Design review of the part built by this model. Coordinates are the model's own, in mm. Coordinates: 2 decimals unless noted, no trailing zeros. Write each loop counter-clockwise with the first axis right and the second up, starting at its lowest first coordinate (ties: lowest second). Pieces come first, ordered by that corner, then holes.
Q1. Take a section at A-A (y = 0). Give the boundary of the cut face in (x, z) (3 decimals), and give its area (3 significant figures).
Q2. For probe 1 along Z at (x, y) = (4.1, 0) (3 decimals); probe 2 along Y at (x, z) = (-1.75, 5.5); probe 3 along Y at (x, z) = (-0.5, 5), list the stretches that pass through material, from the lowest coordinate up.
Q3. Take a section at B-B (z = 9.25). Give the boundary of the cut face in (x, y), and give its area (3 significant figures).
Q4. Insertion check: pin 1 (4 mm diameter, centred on y = 0, z = 6.39, fed in from -X); pin 2 (2 mm diameter, centred on x = -0.5, z = 2.5, fed in from -Y); pin 3 (0.7 mm diameter, centred on x = -0.5, z = 11, fed in from +Y). Each pin has a flat end and moves straight along its axis. Give the tip position at first contact, or say it passes through.
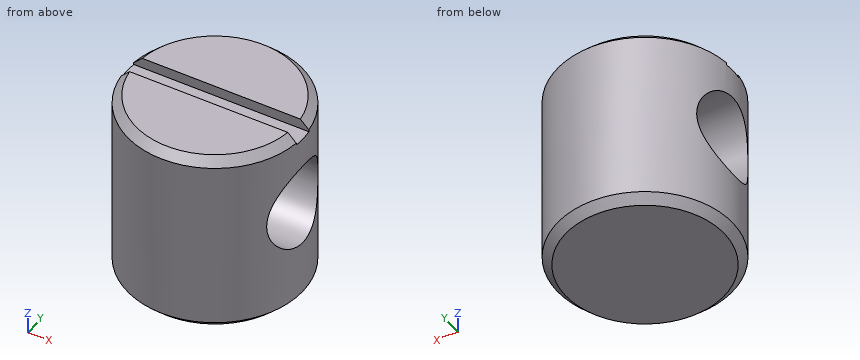
```python
from build123d import *

# Parameters (mm, degrees)
F0_R          = 5.357813
F1_DEPTH      = 11.43
F2_R          = 2.579688
F3_DEPTH      = 25.4
F3_DEPTH_BACK = 25.4
F5_DEPTH      = 0.635
F6_SIZE       = 0.508


with BuildPart() as f1:
    # F0 (on Top) → F1 (new body)
    with BuildSketch(Plane.XY):
        Circle(F0_R)
    extrude(amount=F1_DEPTH)

    # F2 (on Right) → F3 (cut, two sides)
    with BuildSketch(Plane.YZ) as f3_sk:
        with Locations((0, 6.389687)):
            Circle(F2_R)
    extrude(amount=F3_DEPTH, mode=Mode.SUBTRACT)
    extrude(f3_sk.sketch, amount=-F3_DEPTH_BACK, mode=Mode.SUBTRACT)

    # F4 (on face) → F5 (cut)
    with BuildSketch(Plane.XY.offset(11.43)):
        with BuildLine():
            Line((5.32005, 0.635), (-5.32005, 0.635))
            ThreePointArc((-5.32005, 0.635), (-5.379818, 0), (-5.32005, -0.635))
            Line((-5.32005, -0.635), (5.32005, -0.635))
            ThreePointArc((5.32005, -0.635), (5.379818, 0), (5.32005, 0.635))
        make_face()
    extrude(amount=-F5_DEPTH, mode=Mode.SUBTRACT)

    # F6
    f6_edges = [f1.edges().sort_by_distance(p)[0] for p in [
        (0, -5.357813, 11.43),
        (0, 5.357813, 11.43),
        (-5.357813, 0, 0),
    ]]
    chamfer(f6_edges, length=F6_SIZE)


solid = f1.part
```
Response:
1. outline: (-5.358, 0.508) - (-4.85, 0) - (4.85, 0) - (5.358, 0.508) - (5.358, 3.81) - (-5.358, 3.81) - close; (-5.358, 8.969) - (5.358, 8.969) - (5.358, 10.795) - (-5.358, 10.795) - close
1. area: 60.1 mm2
2. probe 1: z = 0 to 3.81, 8.969 to 10.795
2. probe 2: y = -5.06 to -2.42, 2.42 to 5.06
2. probe 3: y = -5.33 to -2.17, 2.17 to 5.33
3. outline: circle Ø10.72 at (0, 0)
3. area: 90.2 mm2
4. pin 1: passes through
4. pin 2: stops at y = -5.36
4. pin 3: stops at y = 5.36
